The listing builds one solid part. Answer for the finished solid, in the listing's coordinates (mm). Round coordinates to 2 decimals unless told otherwise and drop trailing zeros. One line per item, written item: value. Start each with the question number.
1. Straight lines are drawn through the part: line 1 (Z direction, x = 23, y = -14.25); line 2 (Z direction, x = 5.5, y = -2.75). For each, find the intervals that lie inside material, in ascending order.
2. Flat-ended cylindrical pins translate along their axes: P1, Ø8, axis at x = 8, y = -7.5, coming from the -Z side; P2, Ø0.5, axis at x = 19, y = -5.5, coming from the -Z side; P3, Ø0.5, axis at x = 4.5, y = -6.5, coming from the -Z side. Find the tip coordinate at first contact, or state that the pin passes through.
3. Section A-A, the plane z = 0.85 is taken. Count the separate pieces of the cut face and the enclosed holes in it, then the cut area to 3 significant figures.
from build123d import *

# Parameters (mm, degrees)
F1_DEPTH = 16.3


with BuildPart() as f1:
    # F0 (on Front) → F1 (new body)
    with BuildSketch(Plane.XZ):
        Polygon((-3.405686, 0.990338), (-5.235078, 0.990338), (-5.231773, 0.948936), (-4.601518, 0.948936), (-4.317693, 0.678378), (-3.686916, 0.678378), (-3.402381, 0.948936), align=None)
        Polygon((-3.398952, 0.990338), (-3.405686, 0.990338), (-3.402381, 0.948936), align=None)
        Polygon((-1.576294, 0.990338), (-3.398952, 0.990338), (-3.402381, 0.948936), (-2.772126, 0.948936), (-2.4883, 0.678378), (-1.857524, 0.678378), (-1.572988, 0.948936), align=None)
        Polygon((-1.56956, 0.990338), (-1.576294, 0.990338), (-1.572988, 0.948936), align=None)
        Polygon((0.253099, 0.990338), (-1.56956, 0.990338), (-1.572988, 0.948936), (-0.942733, 0.948936), (-0.658908, 0.678378), (-0.028131, 0.678378), (0.256404, 0.948936), align=None)
        Polygon((0.259832, 0.990338), (0.253099, 0.990338), (0.256404, 0.948936), align=None)
        Polygon((2.082491, 0.990338), (0.259832, 0.990338), (0.256404, 0.948936), (0.886659, 0.948936), (1.170484, 0.678378), (1.801261, 0.678378), (2.085796, 0.948936), align=None)
        Polygon((2.089224, 0.990338), (2.082491, 0.990338), (2.085796, 0.948936), align=None)
        Polygon((3.911883, 0.990338), (2.089224, 0.990338), (2.085796, 0.948936), (2.716051, 0.948936), (2.999876, 0.678378), (3.630653, 0.678378), (3.915188, 0.948936), align=None)
        Polygon((3.918617, 0.990338), (3.911883, 0.990338), (3.915188, 0.948936), align=None)
        Polygon((5.741275, 0.990338), (3.918617, 0.990338), (3.915188, 0.948936), (4.545443, 0.948936), (4.829269, 0.678378), (5.460045, 0.678378), (5.744581, 0.948936), align=None)
        Polygon((5.748009, 0.990338), (5.741275, 0.990338), (5.744581, 0.948936), align=None)
        Polygon((7.570668, 0.990338), (5.748009, 0.990338), (5.744581, 0.948936), (6.374836, 0.948936), (6.658661, 0.678378), (7.289438, 0.678378), (7.573973, 0.948936), align=None)
        Polygon((7.577401, 0.990338), (7.570668, 0.990338), (7.573973, 0.948936), align=None)
        Polygon((9.40006, 0.990338), (7.577401, 0.990338), (7.573973, 0.948936), (8.204228, 0.948936), (8.488053, 0.678378), (9.11883, 0.678378), (9.403365, 0.948936), align=None)
        Polygon((9.406793, 0.990338), (9.40006, 0.990338), (9.403365, 0.948936), align=None)
        Polygon((11.229452, 0.990338), (9.406793, 0.990338), (9.403365, 0.948936), (10.03362, 0.948936), (10.317445, 0.678378), (10.948222, 0.678378), (11.232758, 0.948936), align=None)
        Polygon((11.236186, 0.990338), (11.229452, 0.990338), (11.232758, 0.948936), align=None)
        Polygon((13.058844, 0.990338), (11.236186, 0.990338), (11.232758, 0.948936), (11.863013, 0.948936), (12.146838, 0.678378), (12.777615, 0.678378), (13.06215, 0.948936), align=None)
        Polygon((13.065578, 0.990338), (13.058844, 0.990338), (13.06215, 0.948936), align=None)
        Polygon((14.888237, 0.990338), (13.065578, 0.990338), (13.06215, 0.948936), (13.692405, 0.948936), (13.97623, 0.678378), (14.607007, 0.678378), (14.891542, 0.948936), align=None)
        Polygon((14.89497, 0.990338), (14.888237, 0.990338), (14.891542, 0.948936), align=None)
        Polygon((16.717629, 0.990338), (14.89497, 0.990338), (14.891542, 0.948936), (15.521797, 0.948936), (15.805622, 0.678378), (16.436399, 0.678378), (16.720934, 0.948936), align=None)
        Polygon((16.724363, 0.990338), (16.717629, 0.990338), (16.720934, 0.948936), align=None)
        Polygon((18.547021, 0.990338), (16.724363, 0.990338), (16.720934, 0.948936), (17.351189, 0.948936), (17.635015, 0.678378), (18.265791, 0.678378), (18.550327, 0.948936), align=None)
        Polygon((18.553755, 0.990338), (18.547021, 0.990338), (18.550327, 0.948936), align=None)
        Polygon((20.376414, 0.990338), (18.553755, 0.990338), (18.550327, 0.948936), (19.180582, 0.948936), (19.464407, 0.678378), (20.095184, 0.678378), (20.379719, 0.948936), align=None)
        Polygon((20.383147, 0.990338), (20.376414, 0.990338), (20.379719, 0.948936), align=None)
        Polygon((22.205806, 0.990338), (20.383147, 0.990338), (20.379719, 0.948936), (21.009974, 0.948936), (21.293799, 0.678378), (21.924576, 0.678378), (22.209111, 0.948936), align=None)
        Polygon((22.212539, 0.990338), (22.205806, 0.990338), (22.209111, 0.948936), align=None)
        Polygon((24.035198, 0.990338), (22.212539, 0.990338), (22.209111, 0.948936), (22.839366, 0.948936), (23.123191, 0.678378), (23.753968, 0.678378), (24.038504, 0.948936), align=None)
        Polygon((24.041932, 0.990338), (24.035198, 0.990338), (24.038504, 0.948936), align=None)
        Polygon((25.86459, 0.990338), (24.041932, 0.990338), (24.038504, 0.948936), (24.668759, 0.948936), (24.952584, 0.678378), (25.583361, 0.678378), (25.867896, 0.948936), align=None)
        Polygon((25.871324, 0.990338), (25.86459, 0.990338), (25.867896, 0.948936), align=None)
        Polygon((27.693983, 0.990338), (25.871324, 0.990338), (25.867896, 0.948936), (26.498151, 0.948936), (26.781976, 0.678378), (27.412753, 0.678378), (27.697288, 0.948936), align=None)
        Polygon((27.700716, 0.990338), (27.693983, 0.990338), (27.697288, 0.948936), align=None)
        Polygon((29.523375, 0.990338), (27.700716, 0.990338), (27.697288, 0.948936), (28.327543, 0.948936), (28.611368, 0.678378), (29.242145, 0.678378), (29.52668, 0.948936), align=None)
        Polygon((29.530108, 0.990338), (29.523375, 0.990338), (29.52668, 0.948936), align=None)
        Polygon((31.352767, 0.990338), (29.530108, 0.990338), (29.52668, 0.948936), (30.156935, 0.948936), (30.440761, 0.678378), (31.071537, 0.678378), (31.356073, 0.948936), align=None)
        Polygon((31.359501, 0.990338), (31.352767, 0.990338), (31.356073, 0.948936), align=None)
        Polygon((33.18216, 0.990338), (31.359501, 0.990338), (31.356073, 0.948936), (31.986328, 0.948936), (32.270153, 0.678378), (32.90093, 0.678378), (33.185465, 0.948936), align=None)
        Polygon((33.188893, 0.990338), (33.18216, 0.990338), (33.185465, 0.948936), align=None)
        Polygon((35.018285, 0.990338), (33.188893, 0.990338), (33.185465, 0.948936), (33.81572, 0.948936), (34.099545, 0.678378), (34.730322, 0.678378), (35.014857, 0.948936), align=None)
    extrude(amount=F1_DEPTH)


solid = f1.part
Answer list:
1. line 1: z = 0.8 to 0.99
1. line 2: z = 0.72 to 0.99
2. P1: stops at z = 0.68
2. P2: stops at z = 0.88
2. P3: stops at z = 0.75
3. separate pieces: 22
3. enclosed holes: 0
3. area: 355 mm²
